Source: CAD feature listing. Evaluate the final solid. Frame: model axes, mm. Face numbers are marked on the shaded views. A direction names the side the tool comes from. Give positions to 0.01 mm unless a question says otherwise; leave off trailing zeros. Write each loop counter-clockwise with the first axis right and the second up, starting at its lowest first coordinate (ties: lowest second). Pieces come first, ordered by that corner, then holes. Notation, with made-up numbers: (-14, 31.5) -> (31, 31.5) arc R28 ccw to (31, 62.5) -> close; hole circle Ø7 at (63, -19). An arc over 180 degrees is marked (long way). Use one line per item in the form item = value. Start each with the question number.
(1) Set-up query: the marked faces 4, 5 and 6. Return all of +Z, -Z, +X, -X, +Y, -Y with unobstructed straight access to the full face (end or side cutting, diameter ignored); none if empty.
(2) Material intervals for line 1 along X through (y, z) = (-3, 3.55); line 2 along X through (y, z) = (-4, 1.25); line 3 along Y through (x, z) = (31, 3.55), sorted ascending. Write a range as from..to.
(3) First-contact query: P1, Ø3, axis at y = -3, z = 4, coming from the +X side; P2, Ø1.8, axis at y = -4, z = 4.5, coming from the -X side; P3, Ø3.5, axis at x = 3.25, z = 3, coming from the -Y side. Flat tips, straight axial feed; report the tip coordinate or a pass-through.
(4) Cut plane C-C, the plane z = 3. Output: boundary loops of the cut face in (x, y).
(5) Cut plane A-A, the plane x = 36.75. Output: boundary loops of the cut face in (y, z).
(6) Cut plane B-B, the plane y = -3. Output: boundary loops of the cut face in (x, z), and give its area (3 significant figures).
(7) Cut plane D-D, the plane z = 0.95. Output: boundary loops of the cut face in (x, y).
(8) Draft query along Z for the marked faces 1, 2 and 3. Return one class per face: pulls with the +Z half, pulls with the -Z half, needs draft (parallel to the pull), parting line crosses it, or undercut.
Autodesk Fusion 360 part; units mm, degrees
sketch "Sketch1" plane through (0, 0, 0) normal (0, 0, 1) x (1, 0, 0)
  line L0 (0, 0) -> (40, 0)
  line L1 (40, 0) -> (40, 6)
  line L2 (40, 6) -> (0, 6)
  line L3 (0, 6) -> (0, 0)
  dimension "d1" = 40
  dimension "d2" = 6
extrude "Extrude1" add sketch "Sketch1" along normal blind 6
sketch "Sketch2" plane through (0, 0, 0) normal (0, -1, 0) x (1, 0, 0)
  line L0 (0, 0) -> (40, 0)
  line L1 (40, 0) -> (40, 6)
  line L2 (40, 6) -> (0, 6)
  line L3 (0, 6) -> (0, 0)
  line L4 (6.5, 0) -> (33.5, 0)
  line L5 (33.5, 0) -> (33.5, 6)
  line L6 (33.5, 6) -> (6.5, 6)
  line L7 (6.5, 6) -> (6.5, 0)
  dimension "d5" = 27
  dimension "d6" = 6
extrude "Extrude2" add sketch "Sketch2" along normal blind 6 contours L0 L2 L4 L5 L6 L7
hole "Hole1" at (3.25, 0, 3) direction (0, 1, 0) diameter 2.529 depth 6 tip angle 118
hole "Hole2" at (36.75, 0, 3) direction (0, 1, 0) diameter 2.529 depth 6 tip angle 118
hole "Hole3" at (9, -3, 6) direction (0, 0, -1) diameter 2.529 depth 6 tip angle 118
hole "Hole4" at (31, -3, 6) direction (0, 0, -1) diameter 2.529 depth 6 tip angle 118
sketch "Sketch3" plane through (0, 6, 0) normal (0, 1, 0) x (-1, 0, 0)
  circle A0 centre (-36.75, 3) radius 1.2645
  circle A1 centre (-3.25, 3) radius 1.2645
  line L0 (-40, 0) -> (0, 0)
  line L1 (0, 0) -> (0, 6)
  line L2 (0, 6) -> (-40, 6)
  line L3 (-40, 6) -> (-40, 0)
  circle A2 centre (-20, 26) radius 25
  dimension "d29" = 50
sketch "Sketch4" plane through (0, -6, 0) normal (0, -1, 0) x (1, 0, 0)
  line L0 (6.5, 6) -> (6.5, 0)
  line L1 (6.5, 0) -> (33.5, 0)
  line L2 (33.5, 0) -> (33.5, 6)
  line L3 (33.5, 6) -> (6.5, 6)
  circle A0 centre (20, 11.5) radius 10.5
  dimension "d30" = 21
loft "Loft1" cut profiles "Sketch3", "Sketch4" section 1 contours L2 A2 | L2 A2 section 2 contours L3 A0 picked at (23.3871, 12.1316)
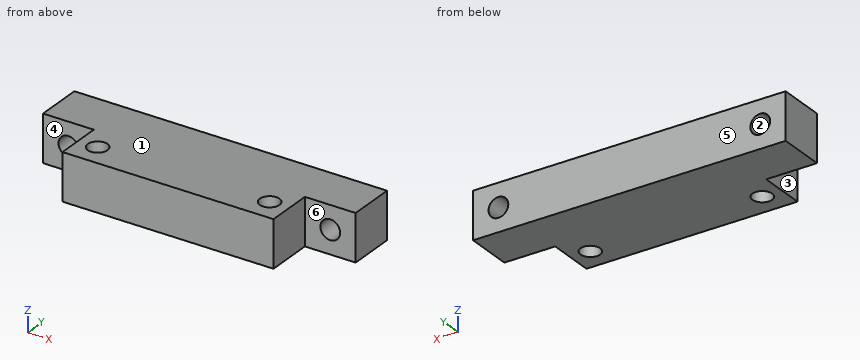
Geometry says:
q1.face_4 = +Z, -Z, -X, -Y
q1.face_5 = +Z, -Z, +X, -X, +Y
q1.face_6 = +Z, -Z, +X, -Y
q2.line_1 = 6.5..7.74, 10.26..29.74, 32.26..33.5
q2.line_2 = 6.5..8.23, 9.77..30.23, 31.77..33.5
q2.line_3 = -6..-4.26, -1.74..6
q3.P1 = 33.5
q3.P2 = 6.5
q3.P3 = 0
q4.outline = (0, 0) -> (1.99, 0) -> (1.99, 6) -> (0, 6) -> close; (4.51, 0) -> (6.5, 0) -> (6.5, -6) -> (33.5, -6) -> (33.5, 0) -> (35.49, 0) -> (35.49, 6) -> (4.51, 6) -> close; (38.01, 0) -> (40, 0) -> (40, 6) -> (38.01, 6) -> close; hole circle Ø2.53 at (9, -3); hole circle Ø2.53 at (31, -3)
q5.outline = (0, 0) -> (6, 0) -> (6, 1.74) -> (0, 1.74) -> close; (0, 4.26) -> (6, 4.26) -> (6, 6) -> (0, 6) -> close
q6.outline = (6.5, 0) -> (7.74, 0) -> (7.74, 6) -> (6.5, 6) -> close; (10.26, 0) -> (29.74, 0) -> (29.74, 6) -> (10.26, 6) -> close; (32.26, 0) -> (33.5, 0) -> (33.5, 6) -> (32.26, 6) -> close
q6.area = 132 mm^2
q7.outline = (0, 0) -> (6.5, 0) -> (6.5, -6) -> (33.5, -6) -> (33.5, 0) -> (40, 0) -> (40, 6) -> (0, 6) -> close; hole circle Ø2.53 at (9, -3); hole circle Ø2.53 at (31, -3)
q8.face_1 = pulls with the +Z half
q8.face_2 = undercut
q8.face_3 = needs draft
